For this review, use the dimensioned drawing (mm, ordinates from the lowest corner) and the shaded views. Give positions to 0.01 mm unless a question says otherwise; leave off trailing zeros. Loops run counter-clockwise (first coordinate to the right, second up) from the corner with the lowest first, then second, coordinate; pieces in that order, holes last. Notation, with made-up numbers: M 55,21 L 91,21 A15 cw 91,33 Z; hole C -13,15.25 d4. An arc over 180 degrees is marked long. Use CSV: the item, a comma, the result in double quotes.
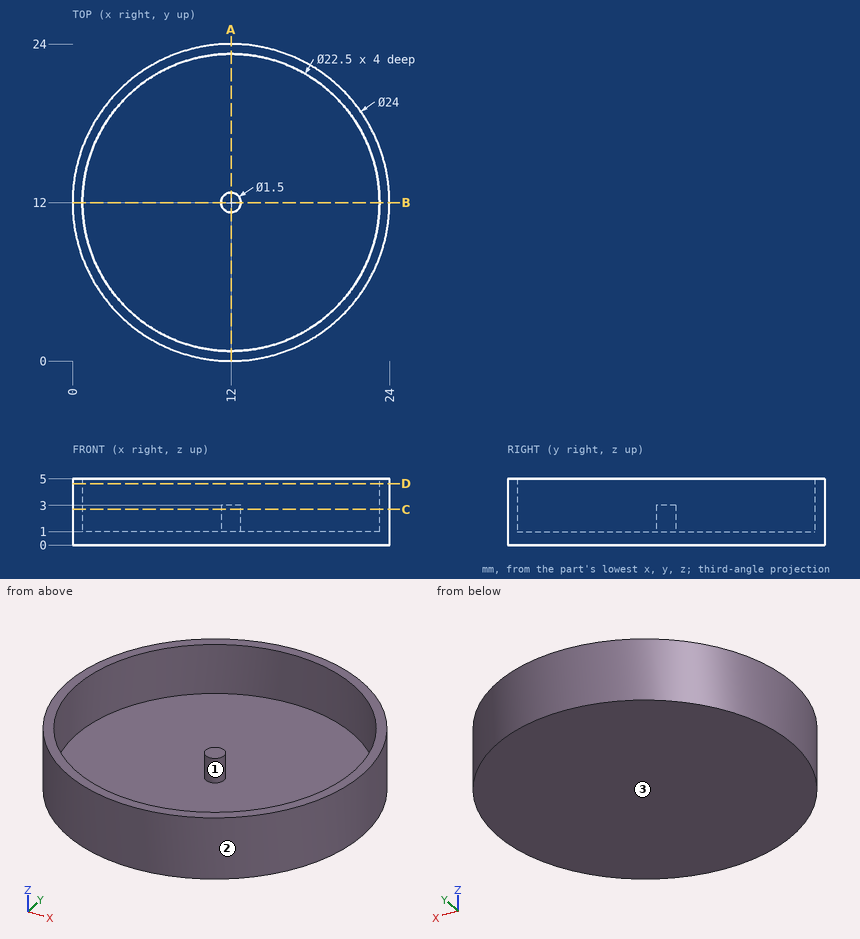
(1) We need section C-C on z = 2.7. State the section outline as (x, y) points, then the cut area to 3 significant figures.
A:
outline,"C 12,12 d24; C 12,12 d1.5; hole C 12,12 d22.5"
area,"56.5 mm²"
(2) We need section D-D on z = 4.65. State the section outline as (x, y) points.
A:
outline,"C 12,12 d24; hole C 12,12 d22.5"
(3) Wall thickness on line 1 along Y through (x, z) = (12, 1.95); line 2 along Y through (x, z) = (12, 3.7); line 3 along Z through (x, y) = (17.75, 10.75): over which ranges is each line inside the solid? List them lowest first. Write a range as [from, to].
A:
line 1,"[0, 0.75], [11.25, 12.75], [23.25, 24]"
line 2,"[0, 0.75], [23.25, 24]"
line 3,"[0, 1]"
(4) The part is to be moulded in two halves that separate along Y. For the marked faces 1, 2 and 3, say which applies: released by +Y, released by -Y, zero draft, split by the parting line, or undercut.
A:
face 1,"undercut"
face 2,"split by the parting line"
face 3,"zero draft"
(5) Clearance check with flat-ended pins moving along their axes: P1, Ø7, axis at x = 16, y = 9.5, coming from the +Z side; P2, Ø13.5, axis at x = 12, y = 12, coming from the +Z side; P3, Ø1, axis at x = 4, z = 2.5, coming from the -Y side. State where each tip first meets the part, or that it passes through.
A:
P1,"z = 1"
P2,"z = 3"
P3,"y = 2.63"
(6) We need section A-A on x = 12. State the section outline as (y, z) points.
A:
outline,"M 0,0 L 24,0 L 24,5 L 23.25,5 L 23.25,1 L 12.75,1 L 12.75,3 L 11.25,3 L 11.25,1 L 0.75,1 L 0.75,5 L 0,5 Z"
